Input: dimensioned drawing with shaded views. Units: mm. Origin: part minimum x, y, z. A direction names the side the tool comes from. Give positions to 0.01 mm unless a question says otherwise; leave off trailing zeros. Order: outer loops, then holes, each group sorted by start corner. A loop starts at its lowest first (then second) coordinate and runs counter-clockwise, first axis right, second up.
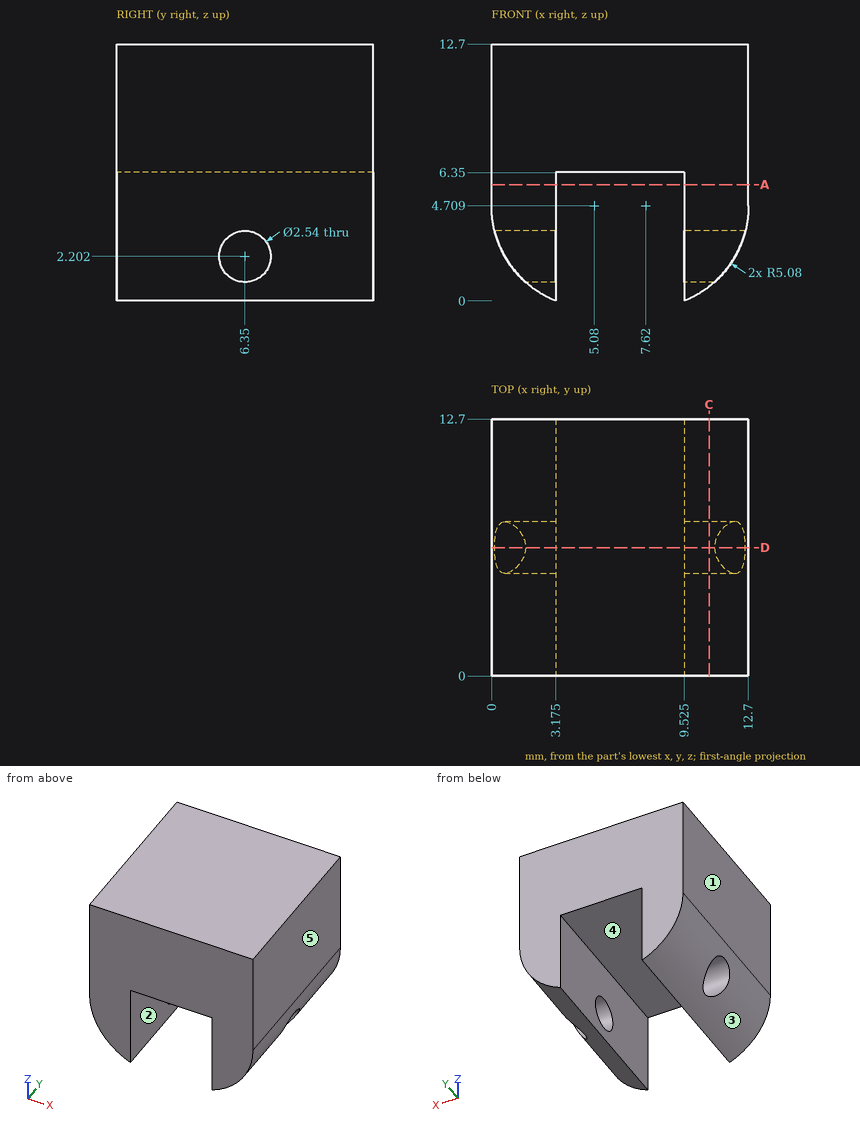
1) Draft query along X for the marked faces 3, 4 and 5. Return one class per face: +X half, -X half, draft (parallel to the pull), parting line (faces both ways), or undercut.
Report:
face 3: -X half
face 4: undercut
face 5: +X half
2) Section query D-D, the plane y = 6.35. Count the separate pieces of the cut face and the enclosed holes in it, and give its area (3 significant figures).
Report:
separate pieces: 3
enclosed holes: 0
area: 100 mm2
3) Pin query (flat end, axial travel): pin 1 (3 mm diameter, centred on x = 2, y = 7, fed in from -Z); pin 2 (3 mm diameter, centred on x = 7.5, y = 5.5, fed in from -Z); pin 3 (5 mm diameter, centred on y = 8, z = 1.5, fed in from +X); pin 4 (4 mm diameter, centred on y = 6.35, z = 2.2, fed in from -X). Return the tip coordinate at first contact, or that it passes through.
Report:
pin 1: stops at z = 0
pin 2: stops at z = 6.35
pin 3: stops at x = 12.65
pin 4: stops at x = 0.03
4) Reachability of the marked faces 1 and 2 from +Z, -Z, +X, -X, +Y, -Y: full face, straight path, thin tool, end or side. Return the list, or none.
Report:
face 1: +Z, -Z, -X, +Y, -Y
face 2: -Z, +Y, -Y
5) Section query A-A, the plane z = 5.75. Return the cut outline in (x, y) (1 decimal).
Report:
outline: (0, 0) - (3.2, 0) - (3.2, 12.7) - (0, 12.7) - close; (9.5, 0) - (12.7, 0) - (12.7, 12.7) - (9.5, 12.7) - close
6) Material intervals for L1, parallel to X at y = 1, z = 5.75 (1 decimal); L2, parallel to Z at x = 0.9, y = 6.35; L3, parallel to Z at x = 6.25, y = 10.5, sorted ascending.
Report:
L1: x = 0 to 3.2, 9.5 to 12.7
L2: z = 3.47 to 12.7
L3: z = 6.35 to 12.7
7) Section query C-C, the plane x = 10.75. Return the cut outline in (y, z), and give its area (3 significant figures).
Report:
outline: (0, 0.71) - (12.7, 0.71) - (12.7, 12.7) - (0, 12.7) - close; hole circle Ø2.54 at (6.35, 2.2)
area: 147 mm2
